The listing builds one solid part. Answer for the finished solid, in the listing's coordinates (mm). Round coordinates to 2 decimals unless told otherwise and drop trailing zeros. Loops run counter-clockwise (first coordinate to the right, second up) from the corner with the lowest first, then second, coordinate; pieces in that order, holes last. Notation, with made-up numbers: M 77,-1 L 109,-1 A24 cw 109,29 Z; hole C 12,40 d10. An arc over 180 degrees is marked long. Answer as a JSON object with one key per item and string values.
```python
from build123d import *

# Parameters (mm, degrees)
F0_R     = 3.175
F1_DEPTH = 152.4
F4_R     = 0.3175
F5_DEPTH = 9.525


with BuildPart() as f1:
    # F0 (on Front) → F1 (new body)
    with BuildSketch(Plane.XZ):
        Circle(F0_R)
    extrude(amount=F1_DEPTH)

    # F2 (on Right) → F3 (revolve)
    with BuildSketch(Plane.YZ):
        with BuildLine():
            Line((-152.4, 0), (-152.4, 3.175))
            ThreePointArc((-152.4, 3.175), (-154.645064, 2.245064), (-155.575, 0))
            Line((-155.575, 0), (-152.4, 0))
        make_face()
    revolve(axis=Axis((0, -168.975449, 0), (0, -1, 0)))

    # F4 (on face) → F5 (join)
    with BuildSketch(Plane(origin=(0, 0, 0), x_dir=(-1, 0, 0), z_dir=(0, 1, 0))):
        with Locations((1.016, -1.016)):
            Circle(F4_R)
        with Locations((-1.016, -1.016)):
            Circle(F4_R)
        with Locations((1.016, 1.016)):
            Circle(F4_R)
        with Locations((-1.016, 1.016)):
            Circle(F4_R)
    extrude(amount=F5_DEPTH)


solid = f1.part
```
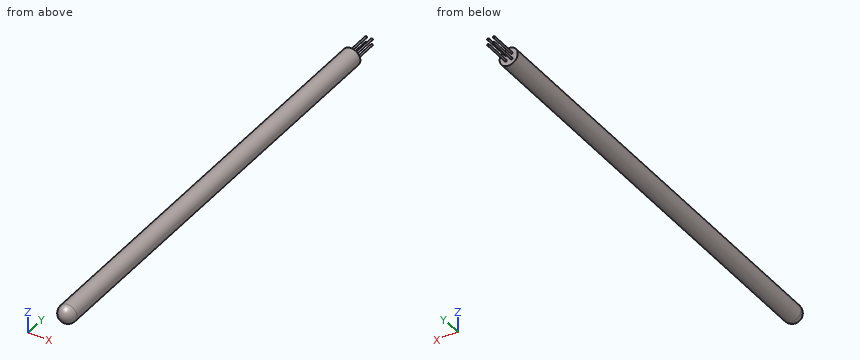
Item 1: Straight lines are drawn through the part: line 1 (Z direction, x = -0.25, y = -68); line 2 (X direction, y = -71.5, z = 2.25). For each, find the intervals that lie inside material, in ascending order.
Values follow:
{"line 1": "-3.17 to 3.17", "line 2": "-2.24 to 2.24"}
Item 2: The part is cut by section A-A (y = -133). Give the vertices of the cut face in (x, z) (3 decimals), then the cut area to 3 significant figures.
Values follow:
{"outline": "C 0,0 d6.35", "area": "31.7 mm^2"}
Item 3: Flat-ended cylindrical pins translate along their axes: P1, Ø1, axis at y = -36.5, z = -2.5, coming from the -X side; P2, Ø1.5, axis at y = -27.5, z = -1, coming from the -X side. Find the tip coordinate at first contact, or state that the pin passes through.
Values follow:
{"P1": "x = -2.47", "P2": "x = -3.17"}
